```python
from build123d import *

# Parameters (mm, degrees)
CYLINDER015_R          = 4
CYLINDER015_DEPTH      = 20
CYLINDER015_ROLL_ANGLE = 90
CYLINDER011_R          = 5
CYLINDER011_DEPTH      = 70
CYLINDER011_ROLL_ANGLE = 90
BOX015_W               = 30
BOX015_H               = 50
BOX015_DEPTH           = 30
FILLET011_R            = 14.8
BOX014_W               = 200
BOX014_H               = 4
BOX014_DEPTH           = 30
BOX014_PITCH_ANGLE     = 90
FILLET010_R            = 14


with BuildPart() as cylindre015:
    # Cylinder015 → Cylinder015 (new body)
    with BuildSketch(Plane.XY):
        Circle(CYLINDER015_R)
    extrude(amount=CYLINDER015_DEPTH)


with BuildPart() as cylindre015_1:
    # Cylinder015 roll: moved
    add(cylindre015.part.rotate(Axis((0, 0, 0), (1, 0, 0)), CYLINDER015_ROLL_ANGLE))


with BuildPart() as cylindre015_2:
    # Cylinder015 placement: moved
    add(cylindre015_1.part.moved(Location((-212, -10, -164))))


with BuildPart() as cylindre011:
    # Cylinder011 → Cylinder011 (new body)
    with BuildSketch(Plane.XY):
        Circle(CYLINDER011_R)
    extrude(amount=CYLINDER011_DEPTH)


with BuildPart() as cylindre011_1:
    # Cylinder011 roll: moved
    add(cylindre011.part.rotate(Axis((0, 0, 0), (1, 0, 0)), CYLINDER011_ROLL_ANGLE))


with BuildPart() as cylindre011_2:
    # Cylinder011 placement: moved
    add(cylindre011_1.part.moved(Location((-210, 37, 4))))


with BuildPart() as fillet011:
    # Box015 → Box015 (new body)
    with BuildSketch(Plane(origin=(-225, -21, -11), x_dir=(1, 0, 0), z_dir=(0, 0, 1))):
        with Locations((15, 25)):
            Rectangle(BOX015_W, BOX015_H)
    extrude(amount=BOX015_DEPTH)

    # Fillet011
    fillet011_edges = [fillet011.edges().sort_by_distance(p)[0] for p in [
        (-225, 4, 19),
        (-225, 4, -11),
        (-195, 4, 19),
        (-195, 4, -11),
    ]]
    fillet(fillet011_edges, radius=FILLET011_R)


with BuildPart() as cut020:
    # Box014 → Box014 (new body)
    with BuildSketch(Plane.XY):
        with Locations((100, 2)):
            Rectangle(BOX014_W, BOX014_H)
    extrude(amount=BOX014_DEPTH)


with BuildPart() as cut020_1:
    # Box014 pitch: moved
    add(cut020.part.rotate(Axis((0, 0, 0), (0, 1, 0)), BOX014_PITCH_ANGLE))


with BuildPart() as cut020_2:
    # Box014 placement: moved
    add(cut020_1.part.moved(Location((-225, -25, 18))))

    # Fillet010
    fillet010_edges = [cut020_2.edges().sort_by_distance(p)[0] for p in [
        (-195, -23, 18),
        (-225, -23, 18),
        (-195, -23, -182),
        (-225, -23, -182),
    ]]
    fillet(fillet010_edges, radius=FILLET010_R)


with BuildPart() as cut020_3:
    # Fillet010 placement: moved
    add(cut020_2.part.moved(Location((0, 0, 1))))

    # Fusion009: union Fillet011
    add(fillet011.part)

    # Cut016: cut Cylindre011
    add(cylindre011_2.part, mode=Mode.SUBTRACT)


with BuildPart() as cut020_4:
    # Cut016 placement: moved
    add(cut020_3.part.moved(Location((-1, 0, 0))))

    # Cut020: cut Cylindre015
    add(cylindre015_2.part, mode=Mode.SUBTRACT)


solid = cut020_4.part
```
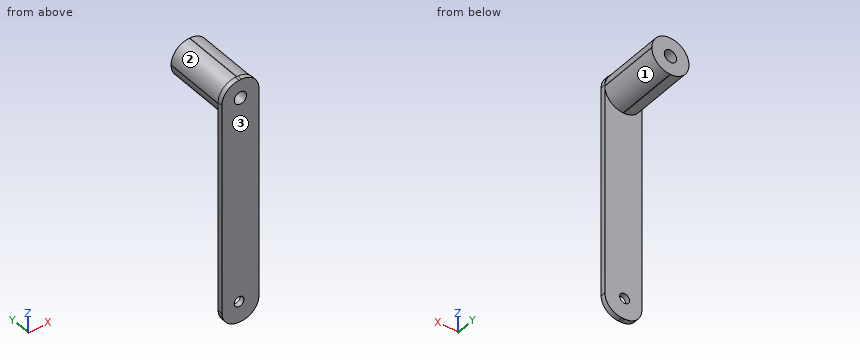
Model file for the job. Use its own axes, mm. Face numbers are marked on the shaded views. A direction names the side the tool comes from. Coordinates: 2 decimals unless noted, no trailing zeros. Write each loop counter-clockwise with the first axis right and the second up, starting at its lowest first coordinate (ties: lowest second). Pieces come first, ordered by that corner, then holes. Notation, with made-up numbers: (36.5, -14.5) - (83.5, -14.5) arc R9 ccw to (83.5, -1.5) - close; hole circle Ø4 at (-12.5, -34.75). An arc over 180 degrees is marked (long way). Use a Markdown table: item, result. Add a question column.
Item 1: Drill centre lines: line 1 along Z through (x, y) = (-212, -23.65); line 2 along X through (y, z) = (-24, -164); line 3 along Z through (x, y) = (-211, -2.5). Where is each one in solid material? Low to high.
Item 2: Band-saw the part on C-C, the plane x = -223.25. Write the cut outline in (y, z).
Item 3: Band-saw the part on D-D, the plane z = -14. Write the cut outline in (x, y), and give its area (3 significant figures).
Item 4: Band-saw the part on A-A, the plane z = -164. Write the cut outline in (x, y), and give its area (3 significant figures).
Item 5: 3-axis set-ups, long thin cutter, end or side, ignore diameter. For the marked faces 1, 2 and 3: which of +Z, -Z, +X, -X, +Y, -Y reach the whole face in a straight line?
Item 6: Band-saw the part on B-B, the plane y = 2. Write the cut outline in (x, z), and give its area (3 significant figures).
Item 7: Drop flat-ended pins along their axis: pin 1 (9 mm diameter, centred on x = -212, z = -164, fed in from +Y); pin 2 (1 mm diameter, centred on x = -201, y = 8.5, fed in from -Z); pin 3 (8 mm diameter, centred on x = -216.5, y = -15.5, fed in from +Z). Give the stop position or say it passes through.
A:
| question | item | result |
|---|---|---|
| 1 | line 1 | z = -181 to -168, -160 to -0.9, 8.9 to 19 |
| 1 | line 2 | x = -226 to -216, -208 to -196 |
| 1 | line 3 | z = -11 to -1, 9 to 19 |
| 2 | outline | (-25, -175.33) - (-21, -175.33) - (-21, -4.79) - (29, -4.79) - (29, 12.79) - (-21, 12.79) - (-21, 13.33) - (-25, 13.33) - close |
| 3 | outline | (-226, -25) - (-196, -25) - (-196, -21) - (-226, -21) - close |
| 3 | area | 120 mm² |
| 4 | outline | (-226, -25) - (-216, -25) - (-216, -21) - (-226, -21) - close; (-208, -25) - (-196, -25) - (-196, -21) - (-208, -21) - close |
| 4 | area | 88.0 mm² |
| 5 | face 1 | -Z, +X, +Y |
| 5 | face 2 | +Z, -X, +Y |
| 5 | face 3 | +Z, -Z, +X, -X, -Y |
| 6 | outline | (-226, 3.8) arc R14.8 ccw to (-211.2, -11) - (-210.8, -11) arc R14.8 ccw to (-196, 3.8) - (-196, 4.2) arc R14.8 ccw to (-210.8, 19) - (-211.2, 19) arc R14.8 ccw to (-226, 4.2) - close; hole circle Ø10 at (-211, 4) |
| 6 | area | 633 mm² |
| 7 | pin 1 | stops at y = -21 |
| 7 | pin 2 | stops at z = -7.71 |
| 7 | pin 3 | stops at z = 18.94 |
